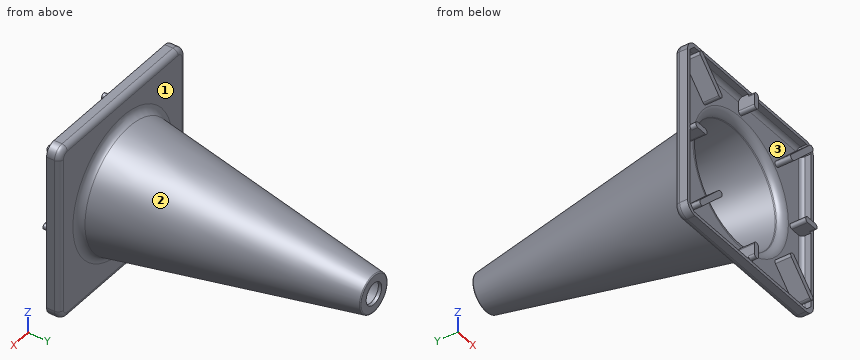
```python
from build123d import *

# Parameters (mm, degrees)
BOSS_EXTRUDE1_DEPTH = 15.875
FILLET1_R           = 6.35
CUT_EXTRUDE1_DEPTH  = 11.90625
BOSS_EXTRUDE2_DEPTH = 11.90625
BOSS_EXTRUDE3_REACH = 25.019
FILLET2_R           = 4.7625


with BuildPart() as part:
    # Sketch1 → Boss-Extrude1 (new body)
    with BuildSketch(Plane(origin=(0, 0, 0), x_dir=(1, 0, 0), z_dir=(0, 1, 0))):
        with BuildLine():
            Line((-93.6625, -106.3625), (93.6625, -106.3625))
            ThreePointArc((93.6625, -106.3625), (102.642756121, -102.642756121), (106.3625, -93.6625))
            Line((106.3625, -93.6625), (106.3625, 93.6625))
            ThreePointArc((106.3625, 93.6625), (102.642756121, 102.642756121), (93.6625, 106.3625))
            Line((93.6625, 106.3625), (-93.6625, 106.3625))
            ThreePointArc((-93.6625, 106.3625), (-102.642756121, 102.642756121), (-106.3625, 93.6625))
            Line((-106.3625, 93.6625), (-106.3625, -93.6625))
            ThreePointArc((-106.3625, -93.6625), (-102.642756121, -102.642756121), (-93.6625, -106.3625))
        make_face()
    extrude(amount=BOSS_EXTRUDE1_DEPTH)

    # Fillet1
    fillet1_edges = [part.edges().sort_by_distance(p)[0] for p in [
        (102.642756121, 15.875, 102.642756121),
        (106.3625, 15.875, 0),
        (102.642756121, 15.875, -102.642756121),
        (0, 15.875, -106.3625),
        (-102.642756121, 15.875, -102.642756121),
        (-106.3625, 15.875, 0),
        (-102.642756121, 15.875, 102.642756121),
        (0, 15.875, 106.3625),
    ]]
    fillet(fillet1_edges, radius=FILLET1_R)

    # Sketch2 → Cut-Extrude1 (cut)
    with BuildSketch(Plane.XZ):
        Polygon((-102.39375, 95.097291902), (-95.097291902, 102.39375), (95.097291902, 102.39375), (102.39375, 95.097291902), (102.39375, -95.097291902), (95.097291902, -102.39375), (-95.097291902, -102.39375), (-102.39375, -95.097291902), align=None)
    extrude(amount=-CUT_EXTRUDE1_DEPTH, mode=Mode.SUBTRACT)

    # Sketch3 → Boss-Extrude2 (add)
    with BuildSketch(Plane.XZ.offset(-11.90625)):
        with BuildLine():
            Line((-3.3734375, 102.39375), (-3.3734375, 86.7171875))
            ThreePointArc((-3.3734375, 86.7171875), (0, 83.34375), (3.3734375, 86.7171875))
            Line((3.3734375, 86.7171875), (3.3734375, 102.39375))
            Line((3.3734375, 102.39375), (-3.3734375, 102.39375))
        make_face()
        with BuildLine():
            Line((102.39375, -3.3734375), (86.7171875, -3.3734375))
            ThreePointArc((86.7171875, -3.3734375), (83.34375, 0), (86.7171875, 3.3734375))
            Line((86.7171875, 3.3734375), (102.39375, 3.3734375))
            Line((102.39375, 3.3734375), (102.39375, -3.3734375))
        make_face()
        with BuildLine():
            Line((-3.3734375, -102.39375), (-3.3734375, -86.7171875))
            ThreePointArc((-3.3734375, -86.7171875), (0, -83.34375), (3.3734375, -86.7171875))
            Line((3.3734375, -86.7171875), (3.3734375, -102.39375))
            Line((3.3734375, -102.39375), (-3.3734375, -102.39375))
        make_face()
        with BuildLine():
            Line((-102.39375, 3.3734375), (-86.7171875, 3.3734375))
            ThreePointArc((-86.7171875, 3.3734375), (-83.34375, 0), (-86.7171875, -3.3734375))
            Line((-86.7171875, -3.3734375), (-102.39375, -3.3734375))
            Line((-102.39375, -3.3734375), (-102.39375, 3.3734375))
        make_face()
    extrude(amount=BOSS_EXTRUDE2_DEPTH)

    # Sketch4 → Boss-Extrude3 (add, up to next)
    with BuildSketch(Plane(origin=(0, -7.14375, 0), x_dir=(-1, 0, 0), z_dir=(0, -1, 0)), mode=Mode.PRIVATE) as boss_extrude3_sk1:
        with BuildLine():
            Line((-94.816658898, 90.045897834), (-63.666395478, 58.895634414))
            ThreePointArc((-63.666395478, 58.895634414), (-58.895634414, 58.895634414), (-58.895634414, 63.666395478))
            Line((-58.895634414, 63.666395478), (-90.045897834, 94.816658898))
            ThreePointArc((-90.045897834, 94.816658898), (-94.816658898, 94.816658898), (-94.816658898, 90.045897834))
        make_face()
    boss_extrude3_tool1 = extrude(boss_extrude3_sk1.sketch, amount=-BOSS_EXTRUDE3_REACH, mode=Mode.PRIVATE) - part.part
    add(boss_extrude3_tool1.solids().sort_by_distance((76.856147, -7.14375, -76.856147))[0])
    # Sketch4 → Boss-Extrude3 (add, up to next)
    with BuildSketch(Plane(origin=(0, -7.14375, 0), x_dir=(-1, 0, 0), z_dir=(0, -1, 0)), mode=Mode.PRIVATE) as boss_extrude3_sk2:
        with BuildLine():
            Line((3.3734375, 86.7171875), (3.3734375, 99.0203125))
            ThreePointArc((3.3734375, 99.0203125), (0, 102.39375), (-3.3734375, 99.0203125))
            Line((-3.3734375, 99.0203125), (-3.3734375, 86.7171875))
            ThreePointArc((-3.3734375, 86.7171875), (0, 83.34375), (3.3734375, 86.7171875))
        make_face()
    boss_extrude3_tool2 = extrude(boss_extrude3_sk2.sketch, amount=-BOSS_EXTRUDE3_REACH, mode=Mode.PRIVATE) - part.part
    add(boss_extrude3_tool2.solids().sort_by_distance((0, -7.14375, -92.86875))[0])
    # Sketch4 → Boss-Extrude3 (add, up to next)
    with BuildSketch(Plane(origin=(0, -7.14375, 0), x_dir=(-1, 0, 0), z_dir=(0, -1, 0)), mode=Mode.PRIVATE) as boss_extrude3_sk3:
        with BuildLine():
            Line((90.045897834, 94.816658898), (58.895634414, 63.666395478))
            ThreePointArc((58.895634414, 63.666395478), (58.895634414, 58.895634414), (63.666395478, 58.895634414))
            Line((63.666395478, 58.895634414), (94.816658898, 90.045897834))
            ThreePointArc((94.816658898, 90.045897834), (94.816658898, 94.816658898), (90.045897834, 94.816658898))
        make_face()
    boss_extrude3_tool3 = extrude(boss_extrude3_sk3.sketch, amount=-BOSS_EXTRUDE3_REACH, mode=Mode.PRIVATE) - part.part
    add(boss_extrude3_tool3.solids().sort_by_distance((-76.856147, -7.14375, -76.856147))[0])
    # Sketch4 → Boss-Extrude3 (add, up to next)
    with BuildSketch(Plane(origin=(0, -7.14375, 0), x_dir=(-1, 0, 0), z_dir=(0, -1, 0)), mode=Mode.PRIVATE) as boss_extrude3_sk4:
        with BuildLine():
            Line((86.7171875, -3.3734375), (99.0203125, -3.3734375))
            ThreePointArc((99.0203125, -3.3734375), (102.39375, 0), (99.0203125, 3.3734375))
            Line((99.0203125, 3.3734375), (86.7171875, 3.3734375))
            ThreePointArc((86.7171875, 3.3734375), (83.34375, 0), (86.7171875, -3.3734375))
        make_face()
    boss_extrude3_tool4 = extrude(boss_extrude3_sk4.sketch, amount=-BOSS_EXTRUDE3_REACH, mode=Mode.PRIVATE) - part.part
    add(boss_extrude3_tool4.solids().sort_by_distance((-92.86875, -7.14375, 0))[0])
    # Sketch4 → Boss-Extrude3 (add, up to next)
    with BuildSketch(Plane(origin=(0, -7.14375, 0), x_dir=(-1, 0, 0), z_dir=(0, -1, 0)), mode=Mode.PRIVATE) as boss_extrude3_sk5:
        with BuildLine():
            Line((94.816658898, -90.045897834), (63.666395478, -58.895634414))
            ThreePointArc((63.666395478, -58.895634414), (58.895634414, -58.895634414), (58.895634414, -63.666395478))
            Line((58.895634414, -63.666395478), (90.045897834, -94.816658898))
            ThreePointArc((90.045897834, -94.816658898), (94.816658898, -94.816658898), (94.816658898, -90.045897834))
        make_face()
    boss_extrude3_tool5 = extrude(boss_extrude3_sk5.sketch, amount=-BOSS_EXTRUDE3_REACH, mode=Mode.PRIVATE) - part.part
    add(boss_extrude3_tool5.solids().sort_by_distance((-76.856147, -7.14375, 76.856147))[0])
    # Sketch4 → Boss-Extrude3 (add, up to next)
    with BuildSketch(Plane(origin=(0, -7.14375, 0), x_dir=(-1, 0, 0), z_dir=(0, -1, 0)), mode=Mode.PRIVATE) as boss_extrude3_sk6:
        with BuildLine():
            Line((-3.3734375, -86.7171875), (-3.3734375, -99.0203125))
            ThreePointArc((-3.3734375, -99.0203125), (0, -102.39375), (3.3734375, -99.0203125))
            Line((3.3734375, -99.0203125), (3.3734375, -86.7171875))
            ThreePointArc((3.3734375, -86.7171875), (0, -83.34375), (-3.3734375, -86.7171875))
        make_face()
    boss_extrude3_tool6 = extrude(boss_extrude3_sk6.sketch, amount=-BOSS_EXTRUDE3_REACH, mode=Mode.PRIVATE) - part.part
    add(boss_extrude3_tool6.solids().sort_by_distance((0, -7.14375, 92.86875))[0])
    # Sketch4 → Boss-Extrude3 (add, up to next)
    with BuildSketch(Plane(origin=(0, -7.14375, 0), x_dir=(-1, 0, 0), z_dir=(0, -1, 0)), mode=Mode.PRIVATE) as boss_extrude3_sk7:
        with BuildLine():
            Line((-90.045897834, -94.816658898), (-58.895634414, -63.666395478))
            ThreePointArc((-58.895634414, -63.666395478), (-58.895634414, -58.895634414), (-63.666395478, -58.895634414))
            Line((-63.666395478, -58.895634414), (-94.816658898, -90.045897834))
            ThreePointArc((-94.816658898, -90.045897834), (-94.816658898, -94.816658898), (-90.045897834, -94.816658898))
        make_face()
    boss_extrude3_tool7 = extrude(boss_extrude3_sk7.sketch, amount=-BOSS_EXTRUDE3_REACH, mode=Mode.PRIVATE) - part.part
    add(boss_extrude3_tool7.solids().sort_by_distance((76.856147, -7.14375, 76.856147))[0])
    # Sketch4 → Boss-Extrude3 (add, up to next)
    with BuildSketch(Plane(origin=(0, -7.14375, 0), x_dir=(-1, 0, 0), z_dir=(0, -1, 0)), mode=Mode.PRIVATE) as boss_extrude3_sk8:
        with BuildLine():
            Line((-86.7171875, 3.3734375), (-99.0203125, 3.3734375))
            ThreePointArc((-99.0203125, 3.3734375), (-102.39375, 0), (-99.0203125, -3.3734375))
            Line((-99.0203125, -3.3734375), (-86.7171875, -3.3734375))
            ThreePointArc((-86.7171875, -3.3734375), (-83.34375, 0), (-86.7171875, 3.3734375))
        make_face()
    boss_extrude3_tool8 = extrude(boss_extrude3_sk8.sketch, amount=-BOSS_EXTRUDE3_REACH, mode=Mode.PRIVATE) - part.part
    add(boss_extrude3_tool8.solids().sort_by_distance((92.86875, -7.14375, 0))[0])

    # Fillet2
    fillet2_edges = [part.edges().sort_by_distance(p)[0] for p in [
        (49.235364701, 11.90625, -102.39375),
        (-102.39375, 11.90625, -49.235364701),
        (-102.39375, 11.90625, 49.235364701),
        (-98.745520951, 11.90625, 98.745520951),
        (49.235364701, 11.90625, 102.39375),
        (98.745520951, 11.90625, 98.745520951),
        (102.39375, 11.90625, -49.235364701),
        (98.745520951, 11.90625, -98.745520951),
        (-49.235364701, 11.90625, -102.39375),
        (-98.745520951, 11.90625, -98.745520951),
        (-49.235364701, 11.90625, 102.39375),
        (102.39375, 11.90625, 49.235364701),
    ]]
    fillet(fillet2_edges, radius=FILLET2_R)

    # Sketch5 → Revolve1 (revolve)
    with BuildSketch(Plane.XY):
        with BuildLine():
            Line((74.811263488, 23.744742818), (23.01875, 317.244450958))
            ThreePointArc((23.01875, 317.244450958), (22.584348758, 317.996681194), (21.768073748, 318.29375))
            Line((21.768073748, 318.29375), (13.096875, 318.29375))
            Line((13.096875, 318.29375), (13.096875, 314.325))
            Line((13.096875, 314.325), (19.503862058, 314.325))
            Line((19.503862058, 314.325), (72.169930274, 15.875))
            Line((72.169930274, 15.875), (84.191335378, 15.875))
            ThreePointArc((84.191335378, 15.875), (78.069272803, 18.103016046), (74.811263488, 23.744742818))
        make_face()
    revolve(axis=Axis((0, 0, 0), (0, 1, 0)))

    # Sketch6 → Cut-Revolve1 (revolve, cut)
    with BuildSketch(Plane.XY):
        with BuildLine():
            Line((0, 21.121495212), (71.244105933, 21.121495212))
            Line((71.244105933, 21.121495212), (71.481540414, 19.775992818))
            ThreePointArc((71.481540414, 19.775992818), (74.739549729, 14.134266046), (80.861612304, 11.90625))
            Line((80.861612304, 11.90625), (0, 11.90625))
            Line((0, 11.90625), (0, 21.121495212))
        make_face()
    revolve(axis=Axis((0, 11.90625, 0), (0, 1, 0)), mode=Mode.SUBTRACT)


solid = part.part
```
Geometry: final body of the model. Coordinates: model frame, mm. Face numbers are marked on the shaded views. Round coordinates to 2 decimals unless told otherwise and drop trailing zeros. Write each loop counter-clockwise with the first axis right and the second up, starting at its lowest first coordinate (ties: lowest second). Pieces come first, ordered by that corner, then holes. Notation, with made-up numbers: (77.5, 76) -> (129.5, 76) arc R19 ccw to (129.5, 97) -> close; hole circle Ø8 at (55.5, 24.5). An arc over 180 degrees is marked (long way). Use CSV: the item, a comma, the result in double quotes. Start each with the question number.
Q1. Section B-B (y = 272). Return loops of the section in (x, z).
Q2. First-contact query: pin 1 Ø17 at (y, z) = (4, -97.5) entering from -X; pin 2 Ø1.5 at (y, z) = (53.5, 28) entering from -X; pin 3 Ø5 at (x, z) = (-39, 75.5) entering from -Y; pin 4 Ø3 at (y, z) = (45, 44.5) entering from +X. Flat tips, straight axial feed; report the tip coordinate or a pass-through.
Q3. Line query: L1, parallel to X at y = 317, z = 0; L2, parallel to Y at x = 53, z = -86.5 (3 decimals); L3, parallel to Z at x = 0, y = 316. Output: solid intervals per line, ascending.
Q4. Pull-direction query (X, two-part tool) for the marked faces 1, 2 and 3; classes: pulls with the +X half, pulls with the -X half, needs draft (parallel to the pull), parting line crosses it, or undercut.
Q5. Section A-A (y = 122). Return loops of the section in (x, z), plus the area to 3 significant figures.
Result sheet:
1,outline,"circle Ø62.01 at (0, 0); hole circle Ø53.95 at (0, 0)"
2,pin 1,"x = -106.36"
2,pin 2,"x = -64.03"
2,pin 3,"y = 11.91"
2,pin 4,"x = 56.62"
3,L1,"-23.06 to -13.1, 13.1 to 23.06"
3,L2,"11.906 to 15.875"
3,L3,"-23.24 to -13.1, 13.1 to 23.24"
4,face 1,"needs draft"
4,face 2,"parting line crosses it"
4,face 3,"undercut"
5,outline,"circle Ø114.95 at (0, 0); hole circle Ø106.89 at (0, 0)"
5,area,"1,400 mm²"
